from build123d import *

# Parameters (mm, degrees)
SKETCH_1_R          = 1.5
EXTRUDE_1_DEPTH     = 4
EXTRUDE_2_DEPTH     = 20.84
EXTRUDE_START       = -4
EXTRUDE_3_DEPTH     = 4
SKETCH_8_R          = 1.5
CUT_EXTRUDE_1_DEPTH = 84.097118968


with BuildPart() as part:
    # 草图1 → 凸台-拉伸1 (new body)
    with BuildSketch(Plane.XY):
        with BuildLine():
            Line((-16.110282893, 33.654208826), (-17.814522763, 23.293438272))
            ThreePointArc((-17.814522763, 23.293438272), (-18.179793181, 22.42908037), (-18.899085656, 21.82645661))
            ThreePointArc((-18.899085656, 21.82645661), (-21.337272658, 19.958522776), (-22.891934151, 17.309568206))
            ThreePointArc((-22.891934151, 17.309568206), (-27.990948412, 14.860061819), (-30.440454799, 19.959076079))
            Line((-30.440454799, 19.959076079), (-25.681476272, 33.517536514))
            ThreePointArc((-25.681476272, 33.517536514), (-25.569637864, 34.115664062), (-25.6428361, 34.719738902))
            Line((-25.6428361, 34.719738902), (-29.24172024, 47.558366666))
            ThreePointArc((-29.24172024, 47.558366666), (-29.31581841, 48.075186607), (-29.253628902, 48.593574353))
            Line((-29.253628902, 48.593574353), (-25.108232608, 64.808221419))
            ThreePointArc((-25.108232608, 64.808221419), (-24.821945701, 65.441071196), (-24.336476636, 65.937839573))
            Line((-24.336476636, 65.937839573), (-12.719407819, 74.272976396))
            ThreePointArc((-12.719407819, 74.272976396), (-12.199607619, 74.311552327), (-11.927927269, 73.866726364))
            Line((-11.927927269, 73.866726364), (-11.927927269, 70.840856193))
            ThreePointArc((-11.927927269, 70.840856193), (-21.765630275, 54.0055336), (-16.519844581, 35.225485153))
            ThreePointArc((-16.519844581, 35.225485153), (-16.148427264, 34.483281689), (-16.110282893, 33.654208826))
        make_face()
        with Locations(Location((-26.666194475, 18.634322143, 0), (0, 0, 180))):
            Circle(SKETCH_1_R, mode=Mode.SUBTRACT)
        with Locations((-21.666194475, 33.634322143)):
            Circle(SKETCH_1_R, mode=Mode.SUBTRACT)
    extrude(amount=EXTRUDE_1_DEPTH)

    # 草图2 → 凸台-拉伸2 (add)
    with BuildSketch(Plane.XY):
        with BuildLine():
            Line((-26.773099146, 38.751829393), (-19.834575078, 40.696814845))
            ThreePointArc((-19.834575078, 40.696814845), (-21.152852216, 57.151552997), (-11.927927269, 70.840856193))
            Line((-11.927927269, 70.840856193), (-11.927927269, 73.866726364))
            ThreePointArc((-11.927927269, 73.866726364), (-12.199607619, 74.311552327), (-12.719407819, 74.272976396))
            Line((-12.719407819, 74.272976396), (-24.336476636, 65.937839573))
            ThreePointArc((-24.336476636, 65.937839573), (-24.821945701, 65.441071196), (-25.108232608, 64.808221419))
            Line((-25.108232608, 64.808221419), (-29.253628902, 48.593574353))
            ThreePointArc((-29.253628902, 48.593574353), (-29.31581841, 48.075186607), (-29.24172024, 47.558366666))
            Line((-29.24172024, 47.558366666), (-26.773099146, 38.751829393))
        make_face()
    extrude(amount=EXTRUDE_2_DEPTH)

    # 草图5 → 凸台-拉伸3 (add)
    with BuildSketch(Plane.XY.offset(20.84).offset(EXTRUDE_START)):
        with BuildLine():
            Line((-19.834575078, 40.696814845), (-26.773099146, 38.751829393))
            Line((-26.773099146, 38.751829393), (-25.6428361, 34.719738902))
            ThreePointArc((-25.6428361, 34.719738902), (-25.569637864, 34.115664062), (-25.681476272, 33.517536514))
            Line((-25.681476272, 33.517536514), (-30.440454799, 19.959076079))
            ThreePointArc((-30.440454799, 19.959076079), (-27.990948412, 14.860061819), (-22.891934151, 17.309568206))
            ThreePointArc((-22.891934151, 17.309568206), (-21.337272658, 19.958522776), (-18.899085656, 21.82645661))
            ThreePointArc((-18.899085656, 21.82645661), (-18.179793181, 22.42908037), (-17.814522763, 23.293438272))
            Line((-17.814522763, 23.293438272), (-16.110282893, 33.654208826))
            ThreePointArc((-16.110282893, 33.654208826), (-16.148427264, 34.483281689), (-16.519844581, 35.225485153))
            ThreePointArc((-16.519844581, 35.225485153), (-18.352935128, 37.854689223), (-19.834575078, 40.696814845))
        make_face()
    extrude(amount=EXTRUDE_3_DEPTH)

    # 草图8 → 切除-拉伸1 (cut, through all)
    with BuildSketch(Plane(origin=(0, 0, 0), x_dir=(-1, 0, 0), z_dir=(0, 0, -1))):
        with Locations(Location((21.666194475, 33.634322143, 0), (0, 0, 180))):
            Circle(SKETCH_8_R)
        with Locations((26.666194475, 18.634322143)):
            Circle(SKETCH_8_R)
    extrude(amount=-CUT_EXTRUDE_1_DEPTH, mode=Mode.SUBTRACT)


solid = part.part
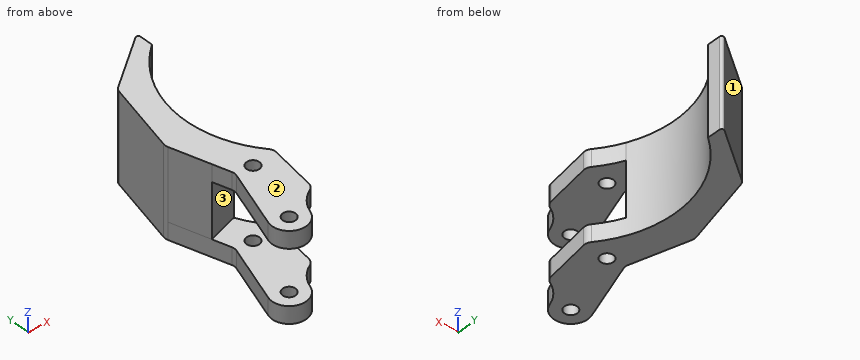
Geometry: final body of the model. Coordinates: model frame, mm. Face numbers are marked on the shaded views. Give positions to 0.01 mm unless a question says otherwise; leave off trailing zeros. Loops run counter-clockwise (first coordinate to the right, second up) from the corner with the lowest first, then second, coordinate; pieces in that order, holes last. Notation, with made-up numbers: M 42.5,34 L 49.5,34 A33 ccw 49.5,70 Z; hole C 44,-6 d4. An arc over 180 degrees is marked long. Put each result on its own line as item: value. Start each with the question number.
1) Cut plane D-D (y = 36.5). Output: boundary loops of the cut face in (x, z), then the cut area to 3 significant figures.
2) Ray query, line 1 along Z through (x, y) = (-23.75, 20); line 2 along Y through (x, z) = (-22.75, 16.5); line 3 along X through (y, z) = (66, 12). Return the intervals inside material, ascending.
3) Pull-direction query (Z, two-part tool) for the marked faces 1, 2 and 3; classes: pulls with the +Z half, pulls with the -Z half, needs draft (parallel to the pull), parting line crosses it, or undercut.
4) Cut plane C-C (z = 17.5). Output: boundary loops of the cut face in (x, y).
5) Contact query for flat-ended pins moving along their axis: pin 1 (4 mm diameter, centred on x = -18.5, z = 7, fed in from -Y); pin 2 (2 mm diameter, centred on x = -19.5, z = 10, fed in from +Y); pin 3 (10 mm diameter, centred on x = -14.5, z = 15, fed in from -Y). Output: stop coordinate, or through.
6) Cut plane B-B (y = 21). Output: boundary loops of the cut face in (x, z), then the cut area to 3 significant figures.
7) Cut plane A-A (z = 7.75). Output: boundary loops of the cut face in (x, y), then the cut area to 3 significant figures.
Verdict:
1. outline: M -26.14,0 L -17.47,0 L -17.47,4 L -26.14,4 Z; M -26.14,16.84 L -17.47,16.84 L -17.47,20.84 L -26.14,20.84 Z
1. area: 69.4 mm2
2. line 1: 0 to 4, 16.84 to 20.84
2. line 2: 39.88 to 67.08
2. line 3: -24.25 to -16.83
3. face 1: needs draft
3. face 2: pulls with the +Z half
3. face 3: undercut
4. outline: M -30.44,19.96 A4 ccw -22.89,17.31 A8 cw -18.9,21.83 A2 ccw -17.81,23.29 L -16.11,33.65 A2 ccw -16.52,35.23 A25 cw -11.93,70.84 L -11.93,73.87 A0.5 ccw -12.72,74.27 L -24.34,65.94 A2 ccw -25.11,64.81 L -29.25,48.59 A2 ccw -29.24,47.56 L -25.64,34.72 A2 cw -25.68,33.52 Z; hole C -26.67,18.63 d3; hole C -21.67,33.63 d3
5. pin 1: y = 40.51
5. pin 2: y = 70.13
5. pin 3: y = 21.7
6. outline: M -30.08,0 L -20.22,0 L -20.22,4 L -30.08,4 Z; M -30.08,16.84 L -20.22,16.84 L -20.22,20.84 L -30.08,20.84 Z
6. area: 78.8 mm2
7. outline: M -29.25,48.59 A2 ccw -29.24,47.56 L -26.77,38.75 L -19.83,40.7 A25 cw -11.93,70.84 L -11.93,73.87 A0.5 ccw -12.72,74.27 L -24.34,65.94 A2 ccw -25.11,64.81 Z
7. area: 219 mm2
